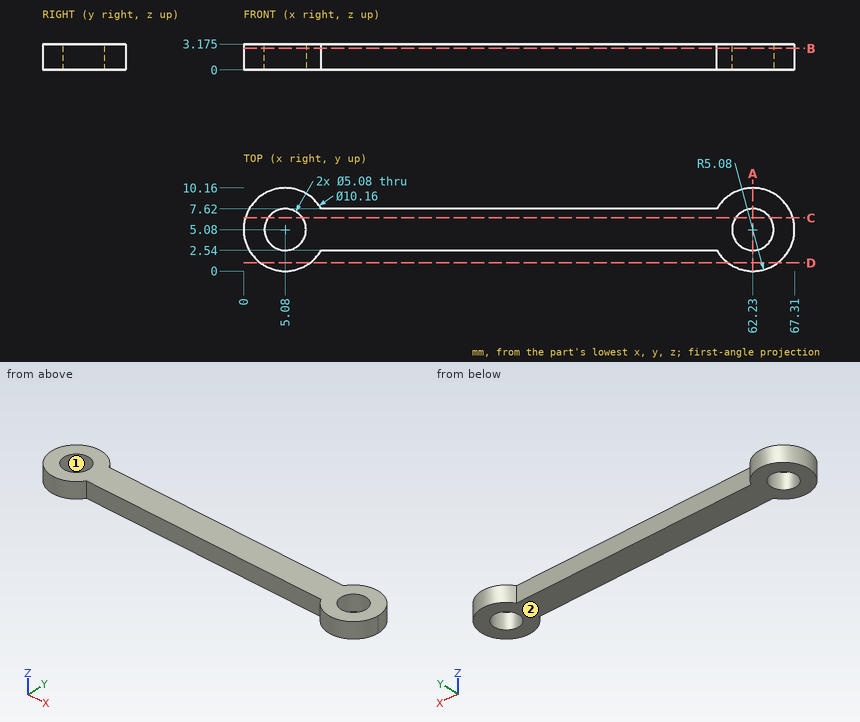
Geometry: see drawing. Coordinates: mm, zero at the bounding-box minimum. Give positions to 0.01 mm unless a question says otherwise; leave off trailing zeros. Loops run counter-clockwise (first coordinate to the right, second up) from the corner with the lowest first, then second, coordinate; pieces in that order, holes last. Notation, with made-up numbers: (37.5, -18) - (57.5, -18) arc R25 ccw to (57.5, 1) - close; hole circle Ø11 at (-24.5, 61.5). An arc over 180 degrees is marked (long way). One line per question, with ' | ' between items. Start each with the question number.
(1) Pull-direction query (X, two-part tool) for the marked faces 1 and 2; classes: released by +X, released by -X, zero draft, split by the parting line, or undercut.
(2) Section query A-A on x = 62.23. Return loops of the section in (y, z) (3 decimals).
(3) Section query C-C on y = 6.5. Return loops of the section in (x, z) (1 decimal).
(4) Contact query for flat-ended pins moving along their axis: pin 1 (1 mm diameter, centred on x = 40.5, z = 2.5, fed in from -Y); pin 2 (4 mm diameter, centred on x = 62.23, y = 5.08, fed in from -Z). Output: stop coordinate, or through.
(5) Section query D-D on y = 1. Return loops of the section in (x, z) (3 decimals), then the cut area to 3 significant figures.
(6) Section query B-B on z = 2.65. Return loops of the section in (x, y).
(7) Ray query, line 1 (Y direction, x = 62.23, z = 1.85); line 2 (X direction, y = 4, z = 2.2); line 3 (X direction, y = 3.5, z = 2.1). Return the intervals inside material, ascending. Write a range as from..to.
The answers:
1) face 1: undercut | face 2: zero draft
2) outline: (0, 0) - (2.54, 0) - (2.54, 3.175) - (0, 3.175) - close; (7.62, 0) - (10.16, 0) - (10.16, 3.175) - (7.62, 3.175) - close
3) outline: (0.2, 0) - (3, 0) - (3, 3.2) - (0.2, 3.2) - close; (7.2, 0) - (60.1, 0) - (60.1, 3.2) - (7.2, 3.2) - close; (64.3, 0) - (67.1, 0) - (67.1, 3.2) - (64.3, 3.2) - close
4) pin 1: y = 2.54 | pin 2: through
5) outline: (2.053, 0) - (8.107, 0) - (8.107, 3.175) - (2.053, 3.175) - close; (59.203, 0) - (65.257, 0) - (65.257, 3.175) - (59.203, 3.175) - close | area: 38.4 mm2
6) outline: (9.48, 2.54) - (57.83, 2.54) arc R5.08 ccw (long way) to (57.83, 7.62) - (9.48, 7.62) arc R5.08 ccw (long way) to start; hole circle Ø5.08 at (5.08, 5.08); hole circle Ø5.08 at (62.23, 5.08)
7) line 1: 0..2.54, 7.62..10.16 | line 2: 0.12..2.78, 7.38..59.93, 64.53..67.19 | line 3: 0.25..3.09, 7.07..60.24, 64.22..67.06
